Source: three-view drawing plus pictorial views. Frame: mm from the lowest corner of the part. A direction names the side the tool comes from. Coordinates: 2 decimals unless noted, no trailing zeros. Loops run counter-clockwise (first coordinate to the right, second up) from the corner with the lowest first, then second, coordinate; pieces in that order, holes last. Notation, with made-up numbers: (58.5, 39.5) - (98.5, 39.5) arc R16 ccw to (98.5, 70.5) - close; hole circle Ø11 at (58.25, 24). An arc over 180 degrees is marked (long way). Return JSON: item names as keys, results as strings.
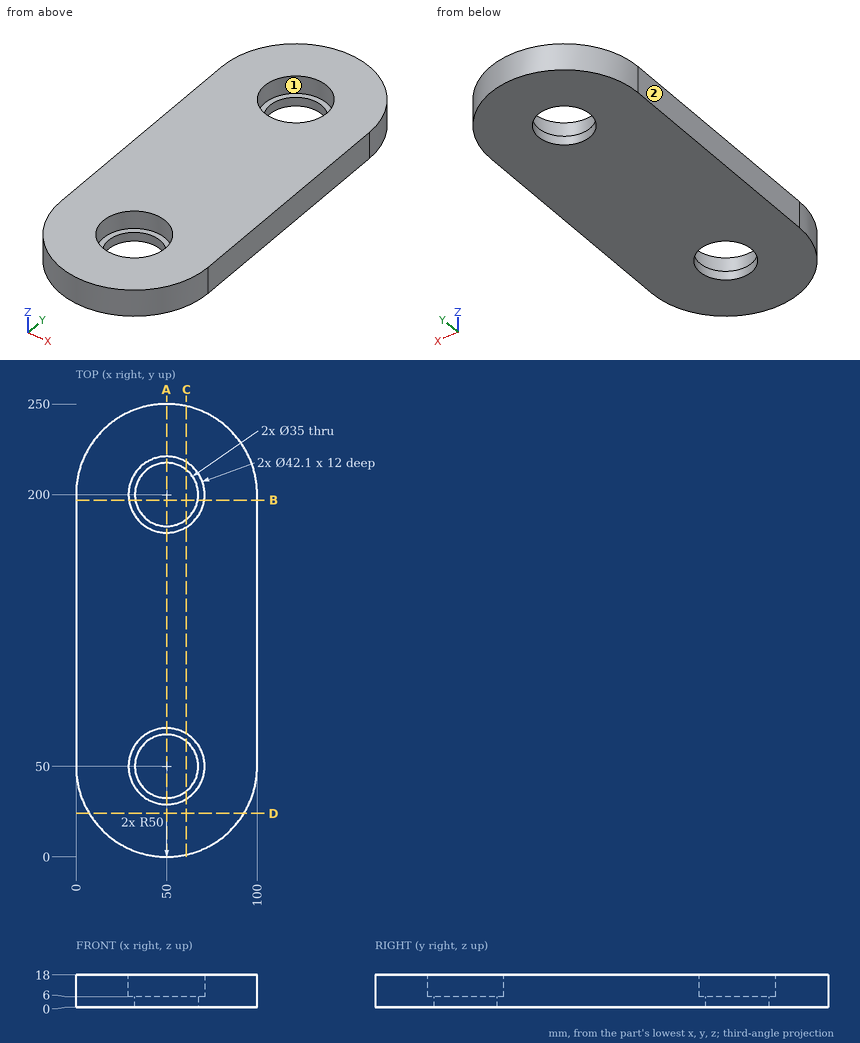
Item 1: Ray query, probe 1 along Y at (x, z) = (49, 13); probe 2 along Y at (x, z) = (50, 1.45); probe 3 along X at (y, z) = (44.5, 7.25). Return the intervals inside material, ascending. Write a range as from..to.
Worked out:
{"probe 1": "0.01..28.97, 71.03..178.97, 221.03..249.99", "probe 2": "0..32.5, 67.5..182.5, 217.5..250", "probe 3": "0.3..29.68, 70.32..99.7"}
Item 2: Section query A-A, the plane x = 50. Return loops of the section in (y, z).
Worked out:
{"outline": "(0, 0) - (32.5, 0) - (32.5, 6) - (28.95, 6) - (28.95, 18) - (0, 18) - close; (67.5, 0) - (182.5, 0) - (182.5, 6) - (178.95, 6) - (178.95, 18) - (71.05, 18) - (71.05, 6) - (67.5, 6) - close; (217.5, 0) - (250, 0) - (250, 18) - (221.05, 18) - (221.05, 6) - (217.5, 6) - close"}
Item 3: First-contact query: pin 1 Ø10 at (y, z) = (33, 2.5) entering from +X; pin 2 Ø4 at (x, z) = (21.5, 15) entering from -Y; pin 3 Ø5 at (x, z) = (86, 14) entering from +Y. Flat tips, straight axial feed; report the tip coordinate or a pass-through.
Worked out:
{"pin 1": "x = 98.54", "pin 2": "y = 7.6", "pin 3": "y = 237.12"}
Item 4: Section query D-D, the plane y = 24. Return loops of the section in (x, z), and give its area (3 significant figures).
Worked out:
{"outline": "(7.29, 0) - (92.71, 0) - (92.71, 18) - (7.29, 18) - close", "area": "1,540 mm^2"}
Item 5: Section query B-B, the plane y = 197. Return loops of the section in (x, z).
Worked out:
{"outline": "(0, 0) - (32.76, 0) - (32.76, 6) - (29.16, 6) - (29.16, 18) - (0, 18) - close; (67.24, 0) - (100, 0) - (100, 18) - (70.84, 18) - (70.84, 6) - (67.24, 6) - close"}
Item 6: Reachability of the marked faces 1 and 2 from +Z, -Z, +X, -X, +Y, -Y: full face, straight path, thin tool, end or side. Return the list, or none.
Worked out:
{"face 1": "+Z", "face 2": "+Z, -Z, -X, +Y, -Y"}
Item 7: Section query C-C, the plane x = 61. Return loops of the section in (y, z) (3 decimals), and give its area (3 significant figures).
Worked out:
{"outline": "(1.225, 0) - (36.389, 0) - (36.389, 6) - (32.053, 6) - (32.053, 18) - (1.225, 18) - close; (63.611, 0) - (186.389, 0) - (186.389, 6) - (182.053, 6) - (182.053, 18) - (67.947, 18) - (67.947, 6) - (63.611, 6) - close; (213.611, 0) - (248.775, 0) - (248.775, 18) - (217.947, 18) - (217.947, 6) - (213.611, 6) - close", "area": "3,270 mm^2"}
